Design review of the part built by this model. Coordinates are the model's own, in mm. Round coordinates to 2 decimals unless told otherwise and drop trailing zeros. Write each loop counter-clockwise with the first axis right and the second up, starting at its lowest first coordinate (ties: lowest second). Pieces come first, ordered by that corner, then holes. Notation, with made-up numbers: (58, -23) -> (67, -23) arc R35 cw to (67, 12) -> close; hole circle Ø3 at (-13.5, -11.75). An arc over 180 degrees is marked (long way). Write item = value, one per line. Start each with the question number.
Item 1: To check wall thickness, follow L1, parallel to Z at x = -708, y = -80.5; L2, parallel to Y at x = -617, z = 56; L3, parallel to Z at x = -1093, y = -96. State the ranges of each line that lie inside material, in increasing order.
Item 2: Add section A-A, the plane x = -364. State the section outline as (y, z) points (3 decimals), then the cut area to 3 significant figures.
Item 3: For pin 1 Ø5 at (x, z) = (-434, -41) entering from +Y, flat-tipped, find the tip position at first contact; note if it passes through.
Item 4: Add section B-B, the plane x = -601.5. State the section outline as (y, z) points (1 decimal).
from build123d import *


with BuildPart() as f1:
    # F0 (on Top) → F1 (revolve)
    with BuildSketch(Plane.XY):
        with BuildLine():
            add(Edge.make_bspline(
                [(0, 0), (-38.4107541448, -6.923547728), (-76.8215082895, -13.847095456), (-114.3, -20.32)],
                knots=[0, 0, 0, 0, 0.145916612, 0.145916612, 0.145916612, 0.145916612], degree=3))
            Line((0, 0), (-114.3, 0))
            Line((-114.3, 0), (-114.3, -20.32))
        make_face()
        with BuildLine():
            Line((0, -17.78), (0, 0))
            add(Edge.make_bspline(
                [(0, 0), (-38.4107541448, -6.923547728), (-76.8215082895, -13.847095456), (-114.3, -20.32)],
                knots=[0, 0, 0, 0, 0.145916612, 0.145916612, 0.145916612, 0.145916612], degree=3))
            Line((-114.3, -20.32), (0, -17.78))
        make_face()
        with BuildLine():
            Line((-114.3, -20.32), (-114.3, 0))
            Line((-114.3, 0), (-215.9, 0))
            Line((-215.9, 0), (-215.9, -38.1))
            add(Edge.make_bspline(
                [(-114.3, -20.32), (-149.6266665218, -26.4212631464), (-184.1250490049, -32.1221448737), (-215.9, -38.1)],
                knots=[0.145916612, 0.145916612, 0.145916612, 0.145916612, 0.2834554311, 0.2834554311, 0.2834554311, 0.2834554311], degree=3))
        make_face()
        with BuildLine():
            Line((-215.9, -38.1), (-114.3, -20.32))
            add(Edge.make_bspline(
                [(-114.3, -20.32), (-149.6266665218, -26.4212631464), (-184.1250490049, -32.1221448737), (-215.9, -38.1)],
                knots=[0.145916612, 0.145916612, 0.145916612, 0.145916612, 0.2834554311, 0.2834554311, 0.2834554311, 0.2834554311], degree=3))
        make_face()
        Polygon((-215.9, -38.1), (-215.9, 0), (-330.2, 0), (-330.2, -57.15), align=None)
        with BuildLine():
            Line((-330.2, -57.15), (-330.2, 0))
            Line((-330.2, 0), (-736.6, 0))
            Line((-736.6, 0), (-736.6, -107.95))
            add(Edge.make_bspline(
                [(-330.2, -57.15), (-424.2035468422, -68.5554317066), (-586.7118007059, -77.9087616289), (-736.6, -107.95)],
                knots=[0.4292365201, 0.4292365201, 0.4292365201, 0.4292365201, 0.7033077599, 0.7033077599, 0.7033077599, 0.7033077599], degree=3))
        make_face()
        with BuildLine():
            Line((-736.6, -107.95), (-330.2, -57.15))
            add(Edge.make_bspline(
                [(-330.2, -57.15), (-424.2035468422, -68.5554317066), (-586.7118007059, -77.9087616289), (-736.6, -107.95)],
                knots=[0.4292365201, 0.4292365201, 0.4292365201, 0.4292365201, 0.7033077599, 0.7033077599, 0.7033077599, 0.7033077599], degree=3))
        make_face()
        with BuildLine():
            Line((-736.6, -107.95), (-736.6, 0))
            Line((-736.6, 0), (-1193.8, 0))
            Line((-1193.8, 0), (-1193.8, -254))
            add(Edge.make_bspline(
                [(-736.6, -107.95), (-898.8595120127, -140.4707501412), (-1046.3297560064, -197.2353750706), (-1193.8, -254)],
                knots=[0.7033077599, 0.7033077599, 0.7033077599, 0.7033077599, 1, 1, 1, 1], degree=3))
        make_face()
    revolve(axis=Axis((-965.2, 0, 0), (-1, 0, 0)))


solid = f1.part
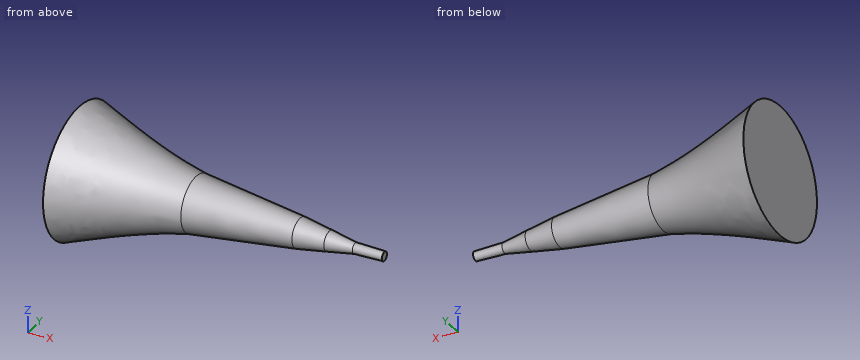
Result set:
q1.L1 = -66.44 to 66.44
q1.L2 = -74.25 to 74.25
q1.L3 = -192.99 to 192.99
q2.outline = circle Ø122.75 at (0, 0)
q2.area = 11,800 mm²
q3.pin_1 = 58.65
q4.outline = circle Ø182.1 at (0, 0)
